```python
from build123d import *

# Parameters (mm, degrees)
CROQUIS1_W        = 247
CROQUIS1_H        = 186
CROQUIS1_W_2      = 243
CROQUIS1_H_2      = 182
WALL_DEPTH        = 24
CROQUIS4_W        = 243
CROQUIS4_H        = 182
FIELD_DEPTH       = 2
CROQUIS5_W        = 219
CROQUIS5_H        = 158
WHITELINE_DEPTH   = 0.01
CROQUIS6_R        = 30
CROQUIS6_R_2      = 29.5
CROQUIS6_R_3      = 1
NEUTRALZONE_DEPTH = 0.1
CROQUIS8_R        = 1
NEUTRALSPOT_DEPTH = 0.1
GOALS_DEPTH       = 10
WEDGE1_DEPTH      = 243
WEDGE2_DEPTH      = 60
WEDGE3_DEPTH      = 60


with BuildPart() as part:
    # Croquis1 → Wall (new body)
    with BuildSketch(Plane(origin=(0, 0, 0), x_dir=(1, 0, 0), z_dir=(0, 1, 0))):
        with Locations((121.5, 91)):
            Rectangle(CROQUIS1_W, CROQUIS1_H)
        with Locations((121.5, 91)):
            Rectangle(CROQUIS1_W_2, CROQUIS1_H_2, mode=Mode.SUBTRACT)
    extrude(amount=WALL_DEPTH)

    # Croquis4 → Field (add)
    with BuildSketch(Plane(origin=(0, 0, 0), x_dir=(1, 0, 0), z_dir=(0, 1, 0))):
        with Locations((121.5, 91)):
            Rectangle(CROQUIS4_W, CROQUIS4_H)
    extrude(amount=FIELD_DEPTH)

    # Croquis5 → WhiteLine (add)
    with BuildSketch(Plane(origin=(0, 2, 0), x_dir=(1, 0, 0), z_dir=(0, 1, 0))):
        with Locations((121.5, 91)):
            Rectangle(CROQUIS5_W, CROQUIS5_H)
        with BuildLine():
            Line((229, 14), (14, 14))
            Line((14, 14), (14, 51))
            Line((14, 51), (24, 51))
            ThreePointArc((24, 51), (34.606601718, 55.393398282), (39, 66))
            Line((39, 66), (39, 91))
            Line((39, 91), (39, 116))
            ThreePointArc((39, 116), (34.606601718, 126.606601718), (24, 131))
            Line((24, 131), (14, 131))
            Line((14, 131), (14, 168))
            Line((14, 168), (229, 168))
            Line((229, 168), (229, 131))
            Line((229, 131), (219, 131))
            ThreePointArc((219, 131), (208.393398282, 126.606601718), (204, 116))
            Line((204, 116), (204, 91))
            Line((204, 91), (204, 66))
            ThreePointArc((204, 66), (208.393398282, 55.393398282), (219, 51))
            Line((219, 51), (229, 51))
            Line((229, 51), (229, 14))
        make_face(mode=Mode.SUBTRACT)
        with BuildLine():
            Line((219, 53), (229, 53))
            Line((229, 53), (229, 129))
            Line((229, 129), (219, 129))
            ThreePointArc((219, 129), (209.807611845, 125.192388155), (206, 116))
            Line((206, 116), (206, 93))
            Line((206, 93), (206, 89))
            Line((206, 89), (206, 66))
            ThreePointArc((206, 66), (209.807611845, 56.807611845), (219, 53))
        make_face(mode=Mode.SUBTRACT)
        with BuildLine():
            Line((24, 129), (14, 129))
            Line((14, 129), (14, 53))
            Line((14, 53), (24, 53))
            ThreePointArc((24, 53), (33.192388155, 56.807611845), (37, 66))
            Line((37, 66), (37, 89))
            Line((37, 89), (37, 93))
            Line((37, 93), (37, 116))
            ThreePointArc((37, 116), (33.192388155, 125.192388155), (24, 129))
        make_face(mode=Mode.SUBTRACT)
    extrude(amount=WHITELINE_DEPTH)

    # Croquis6 → Neutralzone (add)
    # profile 1 of 5: a face of its own
    with BuildSketch(Plane(origin=(0, 2, 0), x_dir=(1, 0, 0), z_dir=(0, 1, 0))):
        with Locations(Location((121.5, 91, 0), (0, 0, 90))):
            Circle(CROQUIS6_R)
        with Locations(Location((121.5, 91, 0), (0, 0, 270))):
            Circle(CROQUIS6_R_2, mode=Mode.SUBTRACT)
    # profile 2 of 5: a face of its own
    with BuildSketch(Plane(origin=(0, 2, 0), x_dir=(1, 0, 0), z_dir=(0, 1, 0))):
        with Locations(Location((57, 130, 0), (0, 0, 90))):
            Circle(CROQUIS6_R_3)
    # profile 3 of 5: a face of its own
    with BuildSketch(Plane(origin=(0, 2, 0), x_dir=(1, 0, 0), z_dir=(0, 1, 0))):
        with Locations(Location((57, 52, 0), (0, 0, 90))):
            Circle(CROQUIS6_R_3)
    # profile 4 of 5: a face of its own
    with BuildSketch(Plane(origin=(0, 2, 0), x_dir=(1, 0, 0), z_dir=(0, 1, 0))):
        with Locations(Location((186, 52, 0), (0, 0, 90))):
            Circle(CROQUIS6_R_3)
    # profile 5 of 5: a face of its own
    with BuildSketch(Plane(origin=(0, 2, 0), x_dir=(1, 0, 0), z_dir=(0, 1, 0))):
        with Locations(Location((186, 130, 0), (0, 0, 90))):
            Circle(CROQUIS6_R_3)
    extrude(amount=NEUTRALZONE_DEPTH)

    # Croquis8 → NeutralSpot (add)
    with BuildSketch(Plane(origin=(0, 2, 0), x_dir=(1, 0, 0), z_dir=(0, 1, 0))):
        with Locations(Location((121.5, 91, 0), (0, 0, 90))):
            Circle(CROQUIS8_R)
    extrude(amount=NEUTRALSPOT_DEPTH)

    # Croquis9 → Goals (add)
    with BuildSketch(Plane(origin=(0, 2, 0), x_dir=(1, 0, 0), z_dir=(0, 1, 0))):
        Polygon((14, 121), (6.6, 121), (6.6, 91), (6.6, 61), (14, 61), (14, 60), (5.6, 60), (0, 60), (0, 61), (5.6, 61), (5.6, 91), (5.6, 121), (0, 121), (0, 122), (5.6, 122), (14, 122), align=None)
        Polygon((229, 61), (236.4, 61), (236.4, 91), (236.4, 121), (229, 121), (229, 122), (237.4, 122), (243, 122), (243, 121), (237.4, 121), (237.4, 91), (237.4, 61), (243, 61), (243, 60), (237.4, 60), (229, 60), align=None)
    extrude(amount=GOALS_DEPTH)

    # Croquis10 → Wedge1 (add)
    with BuildSketch(Plane(origin=(0, 0, 0), x_dir=(0, 0, -1), z_dir=(1, 0, 0))):
        Polygon((0, 2), (10, 2), (0, 4), align=None)
        Polygon((182, 4), (172, 2), (182, 2), align=None)
    extrude(amount=WEDGE1_DEPTH)

    # Croquis11 → Wedge2 (add)
    with BuildSketch(Plane(origin=(0, 0, 0), x_dir=(-1, 0, 0), z_dir=(0, 0, -1))):
        Polygon((0, 4), (0, 2), (-10, 2), align=None)
        Polygon((-233, 2), (-243, 4), (-243, 2), align=None)
    extrude(amount=WEDGE2_DEPTH)

    # Croquis12 → Wedge3 (add)
    with BuildSketch(Plane.XY.offset(-182)):
        Polygon((0, 4), (0, 2), (10, 2), align=None)
        Polygon((233, 2), (243, 4), (243, 2), align=None)
    extrude(amount=WEDGE3_DEPTH)


solid = part.part
```
Read the model definition and answer for the solid it produces. Units are mm, in the model's axes. Give positions to 0.01 mm unless a question says otherwise; leave off trailing zeros. One line per item, written item: value. Start each with the question number.
(1) Straight lines are drawn through the part: L1, parallel to X at y = 14.5, z = -40; L2, parallel to Z at x = 194, y = 22.5; L3, parallel to Y at x = 166.5, z = -130. For each, find the intervals that lie inside material, in ascending order.
(2) Flat-ended cylindrical pins translate along their axes: P1, Ø5, axis at x = 42.5, z = -69, coming from the -Y side; P2, Ø10, axis at x = 139.5, z = -143, coming from the +Y side; P3, Ø6, axis at x = 9, z = -92, coming from the +Y side. Find the tip coordinate at first contact, or state that the pin passes through.
(3) For a pull along X with two mould halves and no side action, classify faces 1 (the flat face through (6.6, 7, -91)), 2 (the flat face through (245, 12, -90)), 3 (the flat face through (120, 12, 2)) as released by +X, released by -X, zero draft, split by the parting line, or undercut.
Taken from the geometry:
1. L1: -2 to 0, 243 to 245
1. L2: -184 to -182, 0 to 2
1. L3: 0 to 2
2. P1: y = 0
2. P2: y = 2
2. P3: y = 12
3. face 1: undercut
3. face 2: released by +X
3. face 3: zero draft
